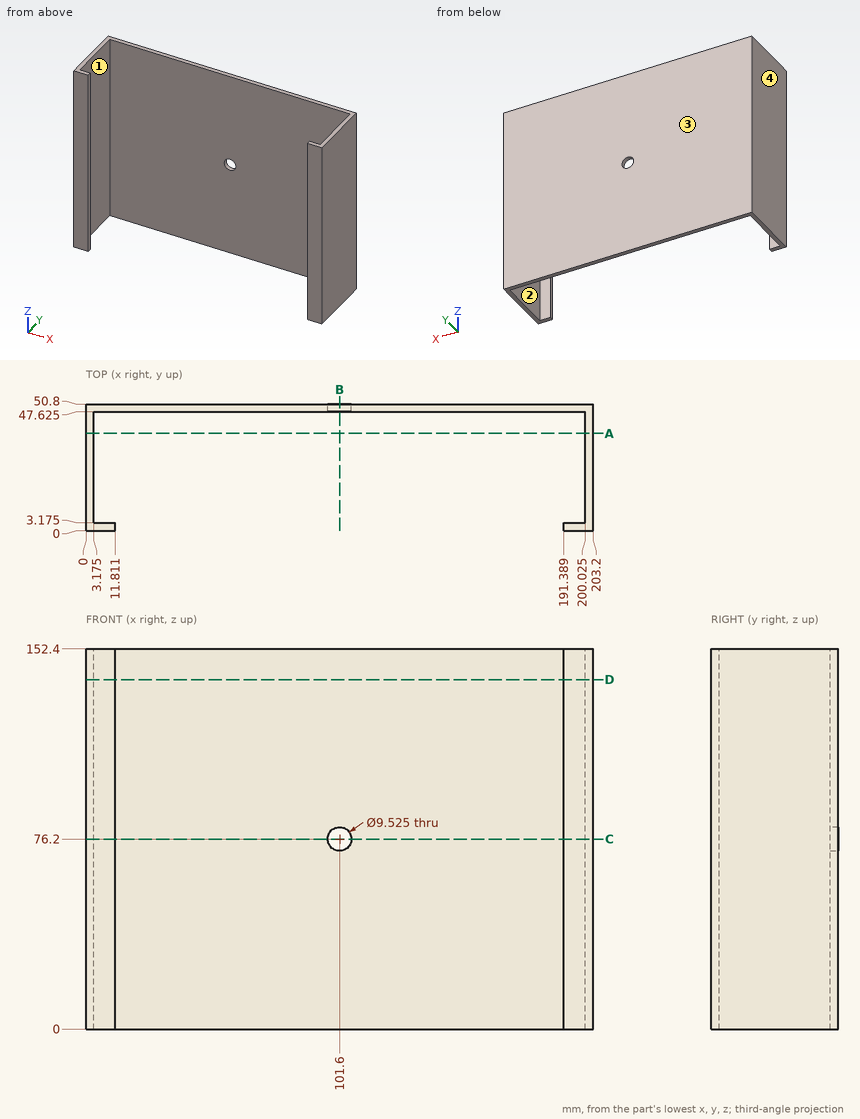
Can you work these out from the drawing? Everything is in mm from the part's minimum corner. Give positions to 0.01 mm unless a question says otherwise; leave off trailing zeros. Loops run counter-clockwise (first coordinate to the right, second up) from the corner with the lowest first, then second, coordinate; pieces in that order, holes last. Notation, with made-up numbers: (80, -29) -> (130, -29) arc R26 cw to (130, 1) -> close; hole circle Ø7 at (49.25, 82). An arc over 180 degrees is marked (long way). Return JSON: item names as keys, results as strings.
Item 1: If we section it at C-C on z = 76.2: List the corners of the cut face in (x, y) for me (1 decimal), plus the area to 3 significant figures.
Geometry results:
{"outline": "(0, 0) -> (11.8, 0) -> (11.8, 3.2) -> (3.2, 3.2) -> (3.2, 47.6) -> (96.8, 47.6) -> (96.8, 50.8) -> (0, 50.8) -> close; (106.4, 47.6) -> (200, 47.6) -> (200, 3.2) -> (191.4, 3.2) -> (191.4, 0) -> (203.2, 0) -> (203.2, 50.8) -> (106.4, 50.8) -> close", "area": "972 mm²"}
Item 2: We'd pull the mould along Y, two halves only. Please class the marked faces 1, 2, 3 and 4: +Y half, -Y half, draft (parallel to the pull), parting line (faces both ways), or undercut.
Geometry results:
{"face 1": "undercut", "face 2": "undercut", "face 3": "+Y half", "face 4": "draft"}
Item 3: I need wall thicknesses on L1, parallel to X at y = 50, z = 76; L2, parallel to X at y = 31.5, z = 41.5 (3 decimals); L3, parallel to Y at x = 175, z = 29.5 (3 decimals). Which ranges of each line are inside material? Lowest first, please. Write a range as from..to.
Geometry results:
{"L1": "x = 0..96.84, 106.36..203.2", "L2": "x = 0..3.175, 200.025..203.2", "L3": "y = 47.625..50.8"}
Item 4: If we section it at B-B on x = 101.6: List the corners of the cut face in (y, z) for me (1 decimal), plus the area to 3 significant figures.
Geometry results:
{"outline": "(47.6, 0) -> (50.8, 0) -> (50.8, 71.4) -> (47.6, 71.4) -> close; (47.6, 81) -> (50.8, 81) -> (50.8, 152.4) -> (47.6, 152.4) -> close", "area": "454 mm²"}
Item 5: If we section it at D-D on z = 140: List the corners of the cut face in (x, y) for me (3 decimals), plus the area to 3 significant figures.
Geometry results:
{"outline": "(0, 0) -> (11.811, 0) -> (11.811, 3.175) -> (3.175, 3.175) -> (3.175, 47.625) -> (200.025, 47.625) -> (200.025, 3.175) -> (191.389, 3.175) -> (191.389, 0) -> (203.2, 0) -> (203.2, 50.8) -> (0, 50.8) -> close", "area": "1,000 mm²"}
Item 6: I'm going to push flat-ended pins straight in: pin 1 (12 mm diameter, centred on x = 182.5, y = 41, fed in from -Z); pin 2 (10 mm diameter, centred on x = 134.5, z = 43, fed in from -Y) (3 decimals); pin 3 (2.5 mm diameter, centred on y = 1, z = 67, fed in from -X). Where does each tip first touch, or does it pass through?
Geometry results:
{"pin 1": "passes through", "pin 2": "stops at y = 47.625", "pin 3": "stops at x = 0"}
Item 7: If we section it at A-A on y = 39: List the corners of the cut face in (x, z) for me (3 decimals), plus the area to 3 significant figures.
Geometry results:
{"outline": "(0, 0) -> (3.175, 0) -> (3.175, 152.4) -> (0, 152.4) -> close; (200.025, 0) -> (203.2, 0) -> (203.2, 152.4) -> (200.025, 152.4) -> close", "area": "968 mm²"}
